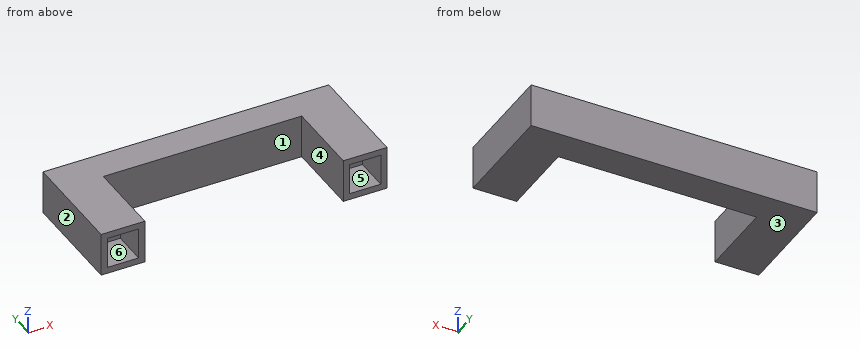
```python
from build123d import *

# Parameters (mm, degrees)
BOSS_EXTRUDE1_DEPTH = 2.8
SKETCH2_W           = 2
SKETCH2_H           = 2
CUT_EXTRUDE1_DEPTH  = 2.2


with BuildPart() as part:
    # Sketch1 → Boss-Extrude1 (new body)
    with BuildSketch(Plane.XY):
        Polygon((0, 0), (0, 7), (18.3, 7), (18.3, 0), (15.5, 0), (15.5, 5), (2.8, 5), (2.8, 0), align=None)
    extrude(amount=BOSS_EXTRUDE1_DEPTH)

    # Sketch2 → Cut-Extrude1 (cut)
    with BuildSketch(Plane.XZ):
        with Locations((16.9, 1.4)):
            Rectangle(SKETCH2_W, SKETCH2_H)
        with Locations((1.4, 1.4)):
            Rectangle(SKETCH2_W, SKETCH2_H)
    extrude(amount=-CUT_EXTRUDE1_DEPTH, mode=Mode.SUBTRACT)


solid = part.part
```
Part model, mm, in its own coordinate system. Face numbers are marked on the shaded views. A direction names the side the tool comes from. Coordinates: 2 decimals unless noted, no trailing zeros. Order: outer loops, then holes, each group sorted by start corner. A loop starts at its lowest first (then second) coordinate and runs counter-clockwise, first axis right, second up. Notation, with made-up numbers: (-35.75, -27.5) -> (-0.75, -27.5) arc R19 ccw to (-0.75, -16.5) -> close; hole circle Ø8 at (-38.75, 36.5). An arc over 180 degrees is marked (long way). Put each result on its own line as item: value. Start each with the question number.
(1) Band-saw the part on A-A (y = 1.25). Give the cut face in (x, z), then the cut area to 3 significant figures.
(2) Band-saw the part on D-D (x = 15). Give the cut face in (y, z), then the cut area to 3 significant figures.
(3) Band-saw the part on C-C (y = 3). Give the cut face in (x, z).
(4) Probe line 1 along X through (y, z) = (0.5, 0.6); line 2 along X through (y, z) = (3.5, 1.15); line 3 along Y through (x, z) = (1, 2.25). List the from-to ranges inside material, lowest first. Write a range as [from, to].
(5) Band-saw the part on B-B (z = 0.85). Give the cut face in (x, y).
(6) Mould opens along Z. For the marked faces 3, 4, 5 and 6 say: pulls with the +Z half, pulls with the -Z half, needs draft (parallel to the pull), parting line crosses it, or undercut.
(7) Pin check, flat tips, straight feed: pin 1 Ø2 at (x, y) = (1, 1) entering from -Z; pin 2 Ø1 at (x, z) = (16.5, 1) entering from -Y; pin 3 Ø1.4 at (x, z) = (11, 2) entering from -Y. Stop position of each tip, or through.
(8) Which spindle directions (+Z, -Z, +X, -X, +Y, -Y) get a long thin tool onto all of the face, cutting with end or side? Do the marked faces 1 and 2. Say none if no direction does.
Determined:
1. outline: (0, 0) -> (2.8, 0) -> (2.8, 2.8) -> (0, 2.8) -> close; (15.5, 0) -> (18.3, 0) -> (18.3, 2.8) -> (15.5, 2.8) -> close; hole (0.4, 0.4) -> (2.4, 0.4) -> (2.4, 2.4) -> (0.4, 2.4) -> close; hole (15.9, 0.4) -> (17.9, 0.4) -> (17.9, 2.4) -> (15.9, 2.4) -> close
1. area: 7.68 mm²
2. outline: (5, 0) -> (7, 0) -> (7, 2.8) -> (5, 2.8) -> close
2. area: 5.60 mm²
3. outline: (0, 0) -> (2.8, 0) -> (2.8, 2.8) -> (0, 2.8) -> close; (15.5, 0) -> (18.3, 0) -> (18.3, 2.8) -> (15.5, 2.8) -> close
4. line 1: x = [0, 0.4], [2.4, 2.8], [15.5, 15.9], [17.9, 18.3]
4. line 2: x = [0, 2.8], [15.5, 18.3]
4. line 3: y = [2.2, 7]
5. outline: (0, 0) -> (0.4, 0) -> (0.4, 2.2) -> (2.4, 2.2) -> (2.4, 0) -> (2.8, 0) -> (2.8, 5) -> (15.5, 5) -> (15.5, 0) -> (15.9, 0) -> (15.9, 2.2) -> (17.9, 2.2) -> (17.9, 0) -> (18.3, 0) -> (18.3, 7) -> (0, 7) -> close
6. face 3: pulls with the -Z half
6. face 4: needs draft
6. face 5: undercut
6. face 6: undercut
7. pin 1: stops at z = 0
7. pin 2: stops at y = 2.2
7. pin 3: stops at y = 5
8. face 1: +Z, -Z, -Y
8. face 2: +Z, -Z, -X, +Y, -Y
